from build123d import *

# Parameters (mm, degrees)
F0_R     = 78
F0_R_2   = 2.375
F0_R_3   = 1.65
F0_R_4   = 63.5
F1_DEPTH = 6.35
F2_R     = 4
F3_DEPTH = 4


# Not quite as in the source:
# - a length typed as a fraction of an inch, garbled in the dataset ("3 / 203.2 mm" for 3/8 in), is restored


with BuildPart() as f1:
    # F0 (on Top) → F1 (new body)
    with BuildSketch(Plane.XY):
        Circle(F0_R)
        with Locations((-35.5625, -61.5960568442)):
            Circle(F0_R_2, mode=Mode.SUBTRACT)
        with Locations((-18.4085045829, -68.7014743948)):
            Circle(F0_R_2, mode=Mode.SUBTRACT)
        with Locations((-68.7014743948, -18.4085045829)):
            Circle(F0_R_2, mode=Mode.SUBTRACT)
        with Locations((0, -75.15)):
            Circle(F0_R_3, mode=Mode.SUBTRACT)
        with Locations((18.4085045829, -68.7014743948)):
            Circle(F0_R_2, mode=Mode.SUBTRACT)
        with Locations((50.2929698119, -50.2929698119)):
            Circle(F0_R_2, mode=Mode.SUBTRACT)
        with Locations((61.5960568442, -35.5625)):
            Circle(F0_R_2, mode=Mode.SUBTRACT)
        with Locations((-75.15, 0)):
            Circle(F0_R_3, mode=Mode.SUBTRACT)
        with Locations((-61.5960568442, 35.5625)):
            Circle(F0_R_2, mode=Mode.SUBTRACT)
        with Locations((-50.2929698119, 50.2929698119)):
            Circle(F0_R_2, mode=Mode.SUBTRACT)
        with Locations((-18.4085045829, 68.7014743948)):
            Circle(F0_R_2, mode=Mode.SUBTRACT)
        Circle(F0_R_4, mode=Mode.SUBTRACT)
        with Locations((75.15, 0)):
            Circle(F0_R_3, mode=Mode.SUBTRACT)
        with Locations((68.7014743948, 18.4085045829)):
            Circle(F0_R_2, mode=Mode.SUBTRACT)
        with Locations((0, 75.15)):
            Circle(F0_R_3, mode=Mode.SUBTRACT)
        with Locations((18.4085045829, 68.7014743948)):
            Circle(F0_R_2, mode=Mode.SUBTRACT)
        with Locations((35.5625, 61.5960568442)):
            Circle(F0_R_2, mode=Mode.SUBTRACT)
    extrude(amount=F1_DEPTH)

    # F2 (on face) → F3 (cut)
    with BuildSketch(Plane.XY.offset(6.35)):
        with Locations((68.7014743948, 18.4085045829)):
            Circle(F2_R)
        with Locations((35.5625, 61.5960568442)):
            Circle(F2_R)
        with Locations((18.4085045829, 68.7014743948)):
            Circle(F2_R)
        with Locations((-18.4085045829, 68.7014743948)):
            Circle(F2_R)
        with Locations((-50.2929698119, 50.2929698119)):
            Circle(F2_R)
        with Locations((-61.5960568442, 35.5625)):
            Circle(F2_R)
        with Locations((-68.7014743948, -18.4085045829)):
            Circle(F2_R)
        with Locations((-35.5625, -61.5960568442)):
            Circle(F2_R)
        with Locations((-18.4085045829, -68.7014743948)):
            Circle(F2_R)
        with Locations((18.4085045829, -68.7014743948)):
            Circle(F2_R)
        with Locations((50.2929698119, -50.2929698119)):
            Circle(F2_R)
        with Locations((61.5960568442, -35.5625)):
            Circle(F2_R)
    extrude(amount=-F3_DEPTH, mode=Mode.SUBTRACT)


solid = f1.part
Source: CAD feature listing. Evaluate the final solid. Frame: model axes, mm. A direction names the side the tool comes from. Round coordinates to 2 decimals unless told otherwise and drop trailing zeros. Loops run counter-clockwise (first coordinate to the right, second up) from the corner with the lowest first, then second, coordinate; pieces in that order, holes last.
Q1. Mould query, pull axis X, two halves, no side actions, for faces 1 (the face through (-10.154, 77.336, 3.131)), 2 (the face through (-52.666, 50.397, 1.159)), 3 (the face through (-12, -63, 0)). Classes: pulls with the +X half, pulls with the -X half, needs draft (parallel to the pull), parting line crosses it, or undercut.
Q2. Section B-B, the plane z = 4.75. State how many separate pieces and enclosed holes the cut face has, plus the area to 3 significant figures.
Q3. Ray query, line 1 (X direction, y = -50, z = 5); line 2 (X direction, y = -37, z = 5); line 3 (X direction, y = 3, z = 3.75). Return the intervals inside material, ascending.
Q4. Section A-A, the plane y = 26. Return loops of the section in (x, z), plus the area to 3 significant figures.
Q5. Access query for faces 4 (the face through (-20.16, -67.1, 1.16)), 5 (the face through (18, 66, 2.35)). Directions: +Z, -Z, +X, -X, +Y, -Y. A direction counts if a zero-diameter tool reaches every point of the face in a straight line with its end or side. Return the directions, or none.
Q6. First-contact query: P1, Ø9, axis at x = 18.41, y = 68.7, coming from the -Z side; P2, Ø1, axis at x = -49, z = 1.5, coming from the -Y side; P3, Ø3, axis at y = 60, z = 5, coming from the +X side; P4, Ø4, axis at x = -16.5, y = -69, coming from the +Z side. Flat tips, straight axial feed; report the tip coordinate or a pass-through.
Solutions:
1. face 1: parting line crosses it
1. face 2: undercut
1. face 3: needs draft
2. separate pieces: 1
2. enclosed holes: 17
2. area: 5,810 mm2
3. line 1: x = -59.87 to -39.14, 39.14 to 46.3, 54.28 to 59.87
3. line 2: x = -68.67 to -51.61, 51.61 to 57.86, 65.33 to 68.67
3. line 3: x = -77.94 to -63.43, 63.43 to 77.94
4. outline: (-73.54, 0) - (-57.93, 0) - (-57.93, 6.35) - (-73.54, 6.35) - close; (57.93, 0) - (73.54, 0) - (73.54, 6.35) - (57.93, 6.35) - close
4. area: 198 mm2
5. face 4: +Z, -Z
5. face 5: +Z
6. P1: stops at z = 0
6. P2: stops at y = -61.09
6. P3: stops at x = 51.59
6. P4: stops at z = 2.35
